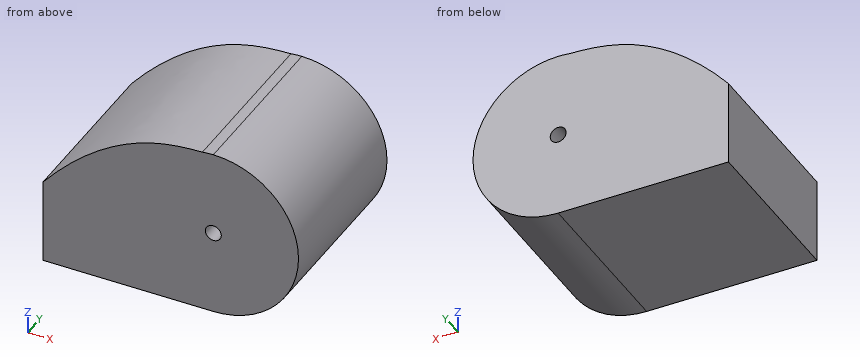
from build123d import *

# Parameters (mm, degrees)
F0_R     = 1.4
F1_DEPTH = 30


with BuildPart() as f1:
    # F0 (on Front) → F1 (new body)
    with BuildSketch(Plane.XZ):
        with BuildLine():
            Line((-30, -15), (0, -15))
            ThreePointArc((0, -15), (15, 0), (0, 15))
            add(Edge.make_bspline(
                [(-1.921847, 14.876374), (-1.200945, 14.903675), (-0.55847, 14.934098), (0, 15)],
                knots=[29.687873, 29.687873, 29.687873, 29.687873, 33.54102, 33.54102, 33.54102, 33.54102], degree=3))
            add(Edge.make_bspline(
                [(-30, 0), (-17.686429, 14.640932), (-7.476277, 14.666022), (-1.921847, 14.876374)],
                knots=[0, 0, 0, 0, 29.687873, 29.687873, 29.687873, 29.687873], degree=3))
            Line((-30, 0), (-30, -15))
        make_face()
        Circle(F0_R, mode=Mode.SUBTRACT)
        with BuildLine():
            add(Edge.make_bspline(
                [(-1.921847, 14.876374), (-1.200945, 14.903675), (-0.55847, 14.934098), (0, 15)],
                knots=[29.687873, 29.687873, 29.687873, 29.687873, 33.54102, 33.54102, 33.54102, 33.54102], degree=3))
            ThreePointArc((0, 15), (-0.962909, 14.969062), (-1.921847, 14.876374))
        make_face()
    extrude(amount=F1_DEPTH)


solid = f1.part
Work out the finished part from the listing and answer in its coordinate system (mm). Coordinates: 2 decimals unless noted, no trailing zeros. Loops run counter-clockwise (first coordinate to the right, second up) from the corner with the lowest first, then second, coordinate; pieces in that order, holes last. Notation, with made-up numbers: M 33.25,75.25 L 58.25,75.25 A7 ccw 58.25,82.25 Z; hole C -3.5,-15 d2. An arc over 180 degrees is marked long. Answer in a Markdown table with one row per item. Add a question column.
1. Consider L1, parallel to X at y = -9.5, z = 0.5; L2, parallel to Z at x = -20.5, y = -2; L3, parallel to Z at x = 11, y = -15.5. Determine where each line is inside the solid, lowest interval first.
2. Flat-ended cylindrical pins translate along their axes: P1, Ø1, axis at y = -10, z = 6.5, coming from the -X side; P2, Ø2, axis at y = -27, z = 5.5, coming from the +X side; P3, Ø1.5, axis at y = -19, z = 6.5, coming from the -X side. Find the tip coordinate at first contact, or state that the pin passes through.
3. Find section B-B, the plane z = -7. Write down the section's boundary in (x, y), then the cut area to 3 significant figures.
4. Find section A-A, the plane x = 7.5. Write down the section's boundary in (y, z), then the cut area to 3 significant figures.
Reported:
| question | item | result |
|---|---|---|
| 1 | L1 | x = -29.58 to -1.31, 1.31 to 14.99 |
| 1 | L2 | z = -15 to 8.98 |
| 1 | L3 | z = -10.2 to 10.2 |
| 2 | P1 | stops at x = -24.22 |
| 2 | P2 | stops at x = 14.31 |
| 2 | P3 | stops at x = -24.5 |
| 3 | outline | M -30,-30 L 13.27,-30 L 13.27,0 L -30,0 Z |
| 3 | area | 1,300 mm^2 |
| 4 | outline | M -30,-12.99 L 0,-12.99 L 0,12.99 L -30,12.99 Z |
| 4 | area | 779 mm^2 |
